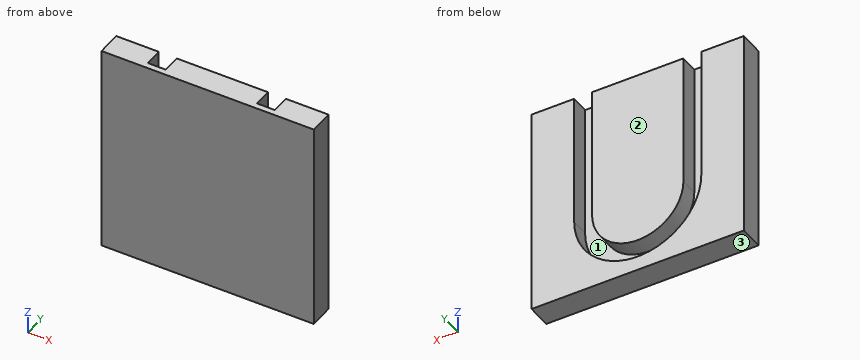
from build123d import *

# Parameters (mm, degrees)
SKETCH1_W           = 35
SKETCH1_H           = 35
BOSS_EXTRUDE1_DEPTH = 1
BOSS_EXTRUDE2_DEPTH = 3


with BuildPart() as part:
    # Sketch1 → Boss-Extrude1 (new body)
    with BuildSketch(Plane(origin=(0, 0, 0), x_dir=(1, 0, 0), z_dir=(0, 1, 0))):
        Rectangle(SKETCH1_W, SKETCH1_H)
    extrude(amount=BOSS_EXTRUDE1_DEPTH)

    # Sketch2 → Boss-Extrude2 (add)
    with BuildSketch(Plane(origin=(0, 1, 0), x_dir=(1, 0, 0), z_dir=(0, 1, 0))):
        with BuildLine():
            Line((-17.5, -17.5), (-10.475, -17.5))
            Line((-10.475, -17.5), (-10.475, 4.65042043))
            ThreePointArc((-10.475, 4.65042043), (0, 15.12542043), (10.475, 4.65042043))
            Line((10.475, 4.65042043), (10.475, -17.5))
            Line((10.475, -17.5), (17.5, -17.5))
            Line((17.5, -17.5), (17.5, 17.5))
            Line((17.5, 17.5), (-17.5, 17.5))
            Line((-17.5, 17.5), (-17.5, -17.5))
        make_face()
        with BuildLine():
            Line((-7.525, 4.65042043), (-7.525, -17.5))
            Line((-7.525, -17.5), (7.525, -17.5))
            Line((7.525, -17.5), (7.525, 4.65042043))
            ThreePointArc((7.525, 4.65042043), (0, 12.17542043), (-7.525, 4.65042043))
        make_face()
    extrude(amount=BOSS_EXTRUDE2_DEPTH)


solid = part.part
Can you work these out from the model? Positions are in its coordinate system, mm. Face numbers are marked on the shaded views. Give positions to 0.01 mm unless a question says otherwise; leave off trailing zeros. Loops run counter-clockwise (first coordinate to the right, second up) from the corner with the lowest first, then second, coordinate; pieces in that order, holes last. Notation, with made-up numbers: M 21.5,63 L 25.5,63 A30 ccw 25.5,88 Z; hole C 35.25,32 d7. An arc over 180 degrees is marked long. One line per item, written item: value. Start each with the question number.
1) If we section it at D-D, the plane z = -14: Write out the boundary of the cut face in (x, y).
2) If we section it at C-C, the plane z = 5.5: Write out the boundary of the cut face in (x, y) (3 decimals).
3) Thinking about a two-plate mould opening in Z: for the marked faces 1, 2 and 3, which applies, +Z half, -Z half, draft (parallel to the pull), parting line (faces both ways), or undercut?
4) If we section it at A-A, the plane y = 2.65: Write out the boundary of the cut face in (x, z) (3 decimals).
5) If we section it at B-B, the plane x = 0: Write out the boundary of the cut face in (y, z).
6) I'm going to push a flat-ended pin straight in: pin 1 (10 mm diameter, centred on x = 10, z = 10.5, fed in from -Y). Where does the tip first touch, or does it pass through?
7) If I drill on line 1 (X direction, y = 1.5, z = 16) (3 decimals); line 2 (X direction, y = 3.4, z = -11.5); line 3 (Y direction, x = -4, z = -12.5), over which ranges is the centre line in solid material (lowest first)? Write a range as [from, to].
Completed:
1. outline: M -17.5,0 L 17.5,0 L 17.5,4 L 4.72,4 L 4.72,1 L -4.72,1 L -4.72,4 L -17.5,4 Z
2. outline: M -17.5,0 L 17.5,0 L 17.5,4 L 10.475,4 L 10.475,1 L 7.525,1 L 7.525,4 L -7.525,4 L -7.525,1 L -10.475,1 L -10.475,4 L -17.5,4 Z
3. face 1: undercut
3. face 2: draft
3. face 3: -Z half
4. outline: M -17.5,-17.5 L 17.5,-17.5 L 17.5,17.5 L 10.475,17.5 L 10.475,-4.65 A10.475 cw -10.475,-4.65 L -10.475,17.5 L -17.5,17.5 Z; M -7.525,-4.65 A7.525 ccw 7.525,-4.65 L 7.525,17.5 L -7.525,17.5 Z
5. outline: M 0,-17.5 L 4,-17.5 L 4,-15.13 L 1,-15.13 L 1,-12.18 L 4,-12.18 L 4,17.5 L 0,17.5 Z
6. pin 1: stops at y = 0
7. line 1: x = [-17.5, -10.475], [-7.525, 7.525], [10.475, 17.5]
7. line 2: x = [-17.5, -7.93], [-3.12, 3.12], [7.93, 17.5]
7. line 3: y = [0, 1]
